Input: dimensioned drawing with shaded views. Units: mm. Origin: part minimum x, y, z. A direction names the side the tool comes from. Coordinates: 2 decimals unless noted, no trailing zeros. Write each loop counter-clockwise with the first axis right and the second up, starting at its lowest first coordinate (ties: lowest second). Pieces come first, ordered by that corner, then holes. Notation, with made-up numbers: M 76.5,51 L 103.5,51 A31 cw 103.5,77 Z; hole C -32,-14.75 d8. An arc over 180 degrees is marked long. Use one line per item in the form item = value.
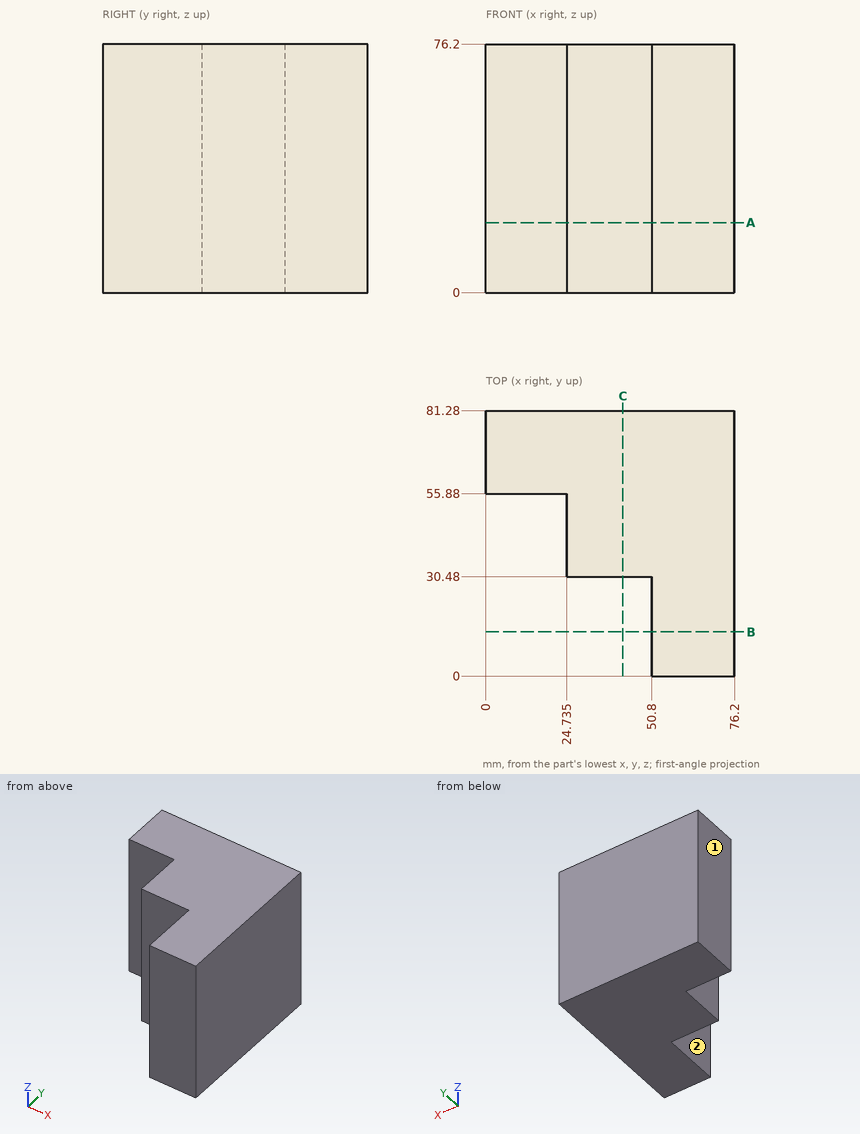
(1) Line query: probe 1 along Y at (x, z) = (47, 12); probe 2 along X at (y, z) = (24, 22.5); probe 3 along Y at (x, z) = (16, 12). Output: solid intervals per line, ascending.
Computed:
probe_1 = 30.48 to 81.28
probe_2 = 50.8 to 76.2
probe_3 = 55.88 to 81.28
(2) Set-up query: the marked faces 1 and 2. Return all of +Z, -Z, +X, -X, +Y, -Y with unobstructed straight access to the full face (end or side cutting, diameter ignored); none if empty.
Computed:
face_1 = +Z, -Z, -X, +Y, -Y
face_2 = +Z, -Z, -X, -Y
(3) Section query B-B on y = 13.5. Return the cut outline in (x, z).
Computed:
outline = M 50.8,0 L 76.2,0 L 76.2,76.2 L 50.8,76.2 Z
(4) Section query C-C on x = 42. Return the cut outline in (y, z).
Computed:
outline = M 30.48,0 L 81.28,0 L 81.28,76.2 L 30.48,76.2 Z
(5) Section query A-A on z = 21.5. Return the cut outline in (x, y) (1 decimal), plus the area to 3 significant figures.
Computed:
outline = M 0,55.9 L 24.7,55.9 L 24.7,30.5 L 50.8,30.5 L 50.8,0 L 76.2,0 L 76.2,81.3 L 0,81.3 Z
area = 4,020 mm^2
(6) First-contact query: pin 1 Ø13 at (x, z) = (32, 45) entering from -Y; pin 2 Ø7.5 at (y, z) = (38, 19.5) entering from -X (1 decimal); pin 3 Ø9 at (y, z) = (10, 39.5) entering from -X. Flat tips, straight axial feed; report the tip coordinate or a pass-through.
Computed:
pin_1 = 30.48
pin_2 = 24.7
pin_3 = 50.8
